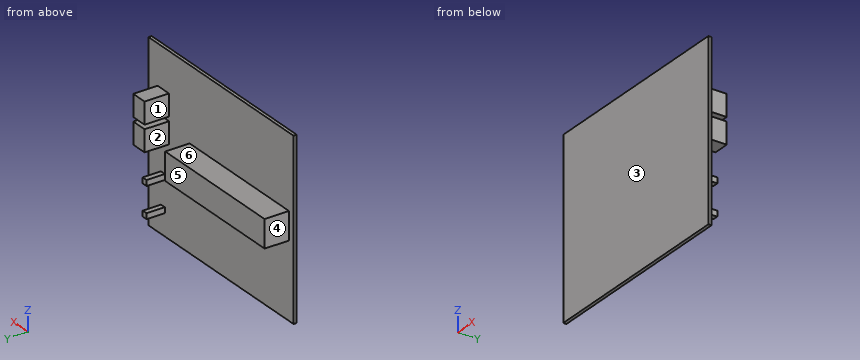
from build123d import *

# Parameters (mm, degrees)
SKETCH3_W           = 102.235
SKETCH3_H           = 86.36
BOSS_EXTRUDE1_DEPTH = 1.56
SKETCH4_W           = 70.061666
SKETCH4_H           = 13.546666
BOSS_EXTRUDE2_DEPTH = 12
SKETCH5_W           = 8
SKETCH5_H           = 10.625667
BOSS_EXTRUDE3_DEPTH = 12
SKETCH6_W           = 2.751667
SKETCH6_H           = 2.751667
BOSS_EXTRUDE4_DEPTH = 9


with BuildPart() as part:
    # Sketch3 → Boss-Extrude1 (new body)
    with BuildSketch(Plane(origin=(0, 0, 0), x_dir=(1, 0, 0), z_dir=(0, 1, 0))):
        with Locations((50.997852632, 42.807288421)):
            Rectangle(SKETCH3_W, SKETCH3_H)
    extrude(amount=BOSS_EXTRUDE1_DEPTH)

    # Sketch4 → Boss-Extrude2 (add)
    with BuildSketch(Plane(origin=(0, 1.56, 0), x_dir=(1, 0, 0), z_dir=(0, 1, 0))):
        with Locations((38.128519632, 42.341621421)):
            Rectangle(SKETCH4_W, SKETCH4_H)
    extrude(amount=BOSS_EXTRUDE2_DEPTH)

    # Sketch5 → Boss-Extrude3 (add)
    with BuildSketch(Plane(origin=(0, 1.56, 0), x_dir=(1, 0, 0), z_dir=(0, 1, 0))):
        with Locations((91.615352632, 37.113454921)):
            Rectangle(SKETCH5_W, SKETCH5_H)
        with Locations((91.615352632, 24.413454921)):
            Rectangle(SKETCH5_W, SKETCH5_H)
    extrude(amount=BOSS_EXTRUDE3_DEPTH)

    # Sketch6 → Boss-Extrude4 (add)
    with BuildSketch(Plane(origin=(0, 1.56, 0), x_dir=(1, 0, 0), z_dir=(0, 1, 0))):
        with Locations((91.934186132, 58.703454921)):
            Rectangle(SKETCH6_W, SKETCH6_H)
        with Locations((91.934186132, 73.943454921)):
            Rectangle(SKETCH6_W, SKETCH6_H)
    extrude(amount=BOSS_EXTRUDE4_DEPTH)


solid = part.part
Design review of the part built by this model. Coordinates are the model's own, in mm. Face numbers are marked on the shaded views. A direction names the side the tool comes from. Coordinates: 2 decimals unless noted, no trailing zeros. Loops run counter-clockwise (first coordinate to the right, second up) from the corner with the lowest first, then second, coordinate; pieces in that order, holes last. Notation, with made-up numbers: (64.5, -35.5) -> (94.5, -35.5) arc R22 ccw to (94.5, -22.5) -> close; hole circle Ø6 at (9, 12). An arc over 180 degrees is marked (long way). Use a Markdown table: item, result. Add a question column.
Item 1: We need section C-C, the plane z = -65. Write out the cut boundary in (x, y), and give its area (3 significant figures).
Item 2: Machinability: for the marked faces 4, 5 and 6, which of the approach directions +Z, -Z, +X, -X, +Y, -Y give a long, thin tool a straight path to every point of the face, cutting with its end or side? Answer none if there is none.
Item 3: We need section D-D, the plane x = 82.5. Write out the cut boundary in (y, z).
Item 4: We need section A-A, the plane y = 9.25. Write out the cut boundary in (x, z), and give its area (3 significant figures).
Item 5: We need section B-B, the plane x = 46. Write out the cut boundary in (y, z), and give its area (3 significant figures).
Item 6: Clearance check with flat-ended pins moving along their axes: P1, Ø1.4, axis at x = 92, y = 7, coming from the -Z side; P2, Ø6, axis at y = 10, z = -43.5, coming from the -X side; P3, Ø0.8, axis at y = 7, z = -73.5, coming from the +X side; P4, Ø4, axis at y = 10.5, z = -52, coming from the -X side. State where each tip first meets the part, or that it passes through.
Item 7: Wall thickness on L1, parallel to Z at x = 94.5, y = 9.5; L2, parallel to Y at x = 69, z = -56.5; L3, parallel to Z at x = 66, y = 3.25: over which ranges is each line inside the solid? List them lowest first. Write a range as from..to.
Item 8: The part is to be moulded in two halves that separate along X. For the marked faces 1, 2 and 3, say which applies: +X half, -X half, draft (parallel to the pull), parting line (faces both ways), or undercut.
Numbers:
| question | item | result |
|---|---|---|
| 1 | outline | (-0.12, 0) -> (102.12, 0) -> (102.12, 1.56) -> (-0.12, 1.56) -> close |
| 1 | area | 159 mm^2 |
| 2 | face 4 | +Z, -Z, -X, +Y |
| 2 | face 5 | +Z, -Z, +X, -X, +Y |
| 2 | face 6 | +Z, -X, +Y |
| 3 | outline | (0, -85.99) -> (1.56, -85.99) -> (1.56, 0.37) -> (0, 0.37) -> close |
| 4 | outline | (3.1, -49.11) -> (73.16, -49.11) -> (73.16, -35.57) -> (3.1, -35.57) -> close; (87.62, -42.43) -> (95.62, -42.43) -> (95.62, -31.8) -> (87.62, -31.8) -> close; (87.62, -29.73) -> (95.62, -29.73) -> (95.62, -19.1) -> (87.62, -19.1) -> close; (90.56, -75.32) -> (93.31, -75.32) -> (93.31, -72.57) -> (90.56, -72.57) -> close; (90.56, -60.08) -> (93.31, -60.08) -> (93.31, -57.33) -> (90.56, -57.33) -> close |
| 4 | area | 1,130 mm^2 |
| 5 | outline | (0, -85.99) -> (1.56, -85.99) -> (1.56, -49.11) -> (13.56, -49.11) -> (13.56, -35.57) -> (1.56, -35.57) -> (1.56, 0.37) -> (0, 0.37) -> close |
| 5 | area | 297 mm^2 |
| 6 | P1 | stops at z = -75.32 |
| 6 | P2 | stops at x = 3.1 |
| 6 | P3 | stops at x = 93.31 |
| 6 | P4 | passes through |
| 7 | L1 | z = -42.43..-31.8, -29.73..-19.1 |
| 7 | L2 | y = 0..1.56 |
| 7 | L3 | z = -49.11..-35.57 |
| 8 | face 1 | -X half |
| 8 | face 2 | undercut |
| 8 | face 3 | draft |
